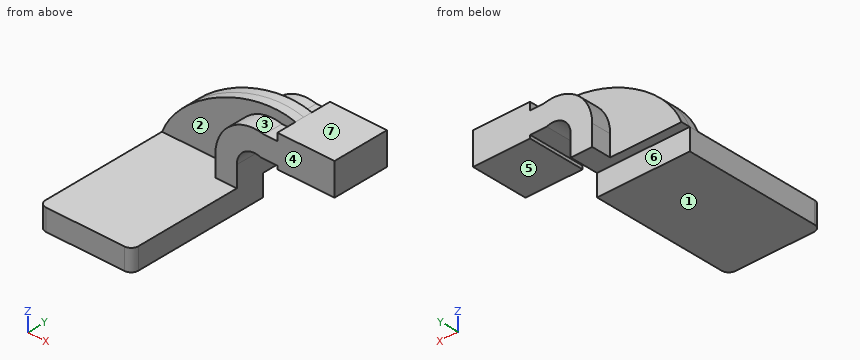
```python
from build123d import *

# Parameters (mm, degrees)
F1_DEPTH = 127
F2_DEPTH = 25.4
F3_DEPTH = 7.9375
F4_R     = 6.35


with BuildPart() as f1:
    # F0 (on Front) → F1 (new body)
    with BuildSketch(Plane.XZ):
        Polygon((-41.275, 9.525), (-41.275, -9.525), (41.275, -9.525), (41.275, 9.525), (22.225, 9.525), align=None)
    extrude(amount=F1_DEPTH)

    # F0 (on Front) → F2 (join, symmetric)
    with BuildSketch(Plane.XZ):
        with BuildLine():
            Line((22.225, 9.525), (41.275, 9.525))
            Line((41.275, 9.525), (41.275, 27.991311))
            ThreePointArc((41.275, 27.991311), (48.084572, 41.023334), (62.671364, 42.8752))
            Line((62.671364, 42.8752), (77.398849, 42.8752))
            Line((77.398849, 42.8752), (77.398849, 61.9252))
            Line((77.398849, 61.9252), (65.411161, 61.9252))
            ThreePointArc((65.411161, 61.9252), (35.571833, 55.45289), (22.225, 27.991311))
            Line((22.225, 27.991311), (22.225, 9.525))
        make_face()
        Polygon((128.198849, 68.58), (77.398849, 68.58), (77.398849, 61.9252), (77.398849, 42.8752), (77.398849, 40.005), (128.198849, 40.005), align=None)
    extrude(amount=F2_DEPTH, both=True)

    # F0 (on Front) → F3 (join, symmetric)
    with BuildSketch(Plane.XZ):
        with BuildLine():
            add(Edge.make_bspline(
                [(-41.275, 9.525), (-25.932714, 48.888751), (38.354626, 80.090507), (77.398849, 68.58)],
                knots=[0, 0, 0, 0, 132.555556, 132.555556, 132.555556, 132.555556], degree=3))
            Line((-41.275, 9.525), (22.225, 9.525))
            Line((22.225, 9.525), (22.225, 27.991311))
            ThreePointArc((22.225, 27.991311), (35.571833, 55.45289), (65.411161, 61.9252))
            Line((65.411161, 61.9252), (77.398849, 61.9252))
            Line((77.398849, 61.9252), (77.398849, 68.58))
        make_face()
    extrude(amount=F3_DEPTH, both=True)

    # F4
    f4_edges = [f1.edges().sort_by_distance(p)[0] for p in [
        (-41.275, -127, 0),
        (41.275, -127, 0),
    ]]
    fillet(f4_edges, radius=F4_R)


solid = f1.part
```
Can you work these out from the model? Positions are in its coordinate system, mm. Face numbers are marked on the shaded views. A direction names the side the tool comes from. Give positions to 0.01 mm unless a question says otherwise; leave off trailing zeros. Write each loop counter-clockwise with the first axis right and the second up, starting at its lowest first coordinate (ties: lowest second). Pieces come first, ordered by that corner, then holes. Notation, with made-up numbers: (23.25, 60) -> (50.25, 60) arc R29 cw to (50.25, 97) -> close; hole circle Ø6 at (26, 46.5). An arc over 180 degrees is marked (long way). Write item = value, one per line.
(1) Suppose I cut it at A-A on y = 13.5. Write out the boundary of the cut face in (x, z) (3 decimals), then the cut area to 3 significant figures.
Worked out:
outline = (22.225, 9.525) -> (41.275, 9.525) -> (41.275, 27.991) arc R15.875 cw to (62.671, 42.875) -> (77.399, 42.875) -> (77.399, 40.005) -> (128.199, 40.005) -> (128.199, 68.58) -> (77.399, 68.58) -> (77.399, 61.925) -> (65.411, 61.925) arc R34.925 ccw to (22.225, 27.991) -> close
area = 2,950 mm^2
(2) Suppose I cut it at B-B on z = 3.5. Write out the boundary of the cut face in (x, y) (3 decimals).
Worked out:
outline = (-41.275, -120.65) arc R6.35 ccw to (-34.925, -127) -> (34.925, -127) arc R6.35 ccw to (41.275, -120.65) -> (41.275, 0) -> (-41.275, 0) -> close
(3) For the marked faces 4, 5, 6 and 7, which set-ups out of +Z, -Z, +X, -X, +Y, -Y let a thin tool reach every point of the face, with its end or its side?
Worked out:
face_4 = +Z, +X, -X, -Y
face_5 = -Z, +X, +Y, -Y
face_6 = -Z, +X, -X, +Y
face_7 = +Z, +X, +Y, -Y
(4) I'm going to push flat-ended pins straight in: P1, Ø4, axis at y = -25.5, z = 30, coming from the +X side; P2, Ø9.5, axis at x = 3, z = -1.5, coming from the +Y side; P3, Ø14, axis at y = -20.5, z = 15, coming from the -X side (3 decimals); P4, Ø2, axis at y = -15.5, z = 66, coming from the -X side. Where does each tip first touch, or does it pass through?
Worked out:
P1 = 41.79
P2 = 0
P3 = -41.275
P4 = 77.4
(5) Suppose I cut it at C-C on x = 91. Write out the boundary of the cut face in (y, z) (3 decimals).
Worked out:
outline = (-25.4, 40.005) -> (25.4, 40.005) -> (25.4, 68.58) -> (-25.4, 68.58) -> close
(6) Thinking about a two-plate mould opening in Z: for the marked faces 1, 2 and 3, which applies, released by +Z, released by -Z, zero draft, split by the parting line, or undercut?
Worked out:
face_1 = released by -Z
face_2 = zero draft
face_3 = released by +Z
(7) I need wall thicknesses on probe 1 along X at (y, z) = (-25, 21) (3 decimals); probe 2 along Z at (x, y) = (86, -20.5) (3 decimals); probe 3 along Y at (x, z) = (82.5, 61.5). Which ranges of each line are inside material? Lowest first, please. Write a range as from..to.
Worked out:
probe_1 = 22.225..41.275
probe_2 = 40.005..68.58
probe_3 = -25.4..25.4
(8) Suppose I cut it at D-D on y = -55. Write out the boundary of the cut face in (x, z) (3 decimals).
Worked out:
outline = (-41.275, -9.525) -> (41.275, -9.525) -> (41.275, 9.525) -> (-41.275, 9.525) -> close
